Geometry: see drawing. Coordinates: mm, zero at the bounding-box minimum. Coordinates: 2 decimals unless noted, no trailing zeros. Write each loop counter-clockwise with the first axis right and the second up, starting at its lowest first coordinate (ties: lowest second). Pieces come first, ordered by that corner, then holes. Notation, with made-up numbers: M -16,-18.75 L 33,-18.75 A31 ccw 33,19.25 Z; hole C -0.5,55.5 d9. An arc over 180 degrees is marked long. Write item = value, one per line. Start each with the question number.
1. Section query D-D (y = 39). Output: boundary loops of the cut face in (x, z).
2. Section query A-A (x = 15.5). Output: boundary loops of the cut face in (y, z).
3. Pin query (flat end, axial travel): pin 1 Ø1.5 at (y, z) = (35, 1) entering from +X; pin 2 Ø0.9 at (x, z) = (1.5, 2) entering from -Y; pin 3 Ø0.9 at (y, z) = (17.5, 2) entering from -X; pin 4 Ø3.5 at (x, y) = (33.5, 39) entering from +Z. Return the tip coordinate at first contact, or that it passes through.
4. Line query: line 1 along Y through (x, z) = (33.5, 1.5); line 2 along Y through (x, z) = (23, 0.95); line 3 along X through (y, z) = (55.5, 0.8). Output: solid intervals per line, ascending.
5. Section query C-C (z = 2.5). Give the number of separate pieces and of enclosed holes in the cut face, then the cut area to 3 significant figures.
6. Section query B-B (y = 15.3). Output: boundary loops of the cut face in (x, z).
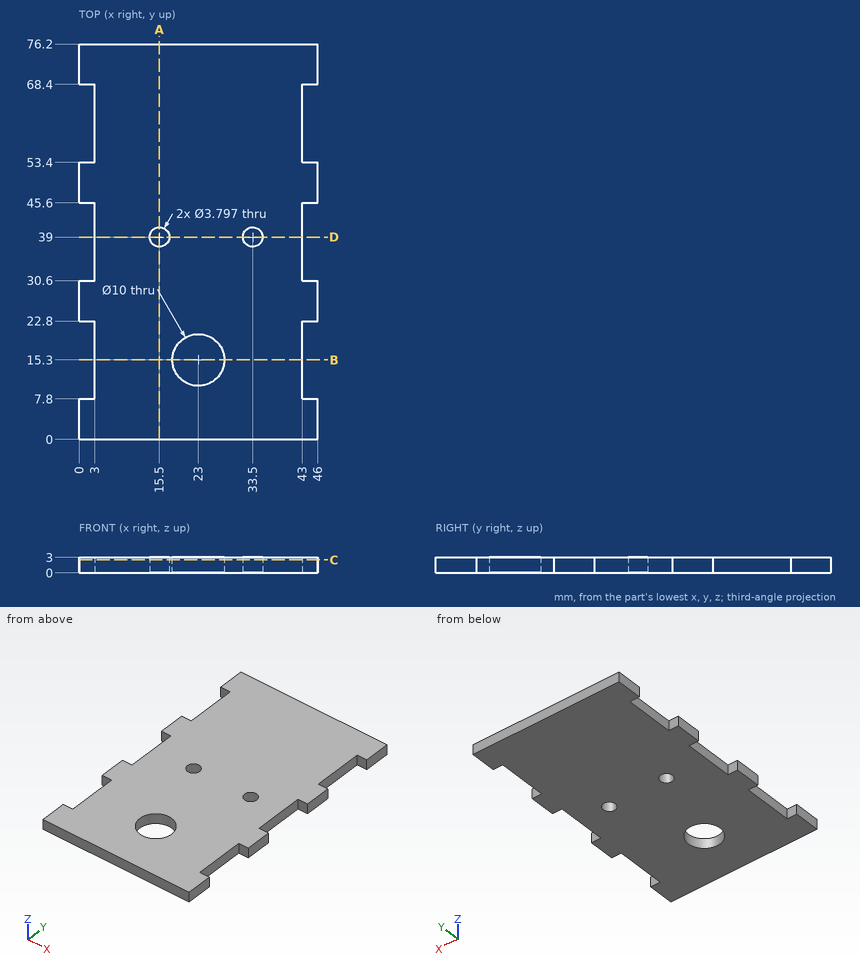
Results are:
q1.outline = M 3,0 L 13.6,0 L 13.6,3 L 3,3 Z; M 17.4,0 L 31.6,0 L 31.6,3 L 17.4,3 Z; M 35.4,0 L 43,0 L 43,3 L 35.4,3 Z
q2.outline = M 0,0 L 37.1,0 L 37.1,3 L 0,3 Z; M 40.9,0 L 76.2,0 L 76.2,3 L 40.9,3 Z
q3.pin_1 = 43
q3.pin_2 = 0
q3.pin_3 = 3
q3.pin_4 = through
q4.line_1 = 0 to 37.1, 40.9 to 76.2
q4.line_2 = 0 to 10.3, 20.3 to 76.2
q4.line_3 = 3 to 43
q5.separate_pieces = 1
q5.enclosed_holes = 3
q5.area = 3,130 mm^2
q6.outline = M 3,0 L 18,0 L 18,3 L 3,3 Z; M 28,0 L 43,0 L 43,3 L 28,3 Z
